Part model, mm, in its own coordinate system. A direction names the side the tool comes from. Round coordinates to 2 decimals unless told otherwise and drop trailing zeros. Write each loop counter-clockwise with the first axis right and the second up, starting at its lowest first coordinate (ties: lowest second). Pieces come first, ordered by that corner, then holes.
1) Which spindle directions (+Z, -Z, +X, -X, +Y, -Y) get a long thin tool onto all of the face, cutting with end or side? Do faces 1 (the cylindrical face through (-5.5, -24.9, 2.5)), 2 (the cylindrical face through (37.24, -20.517, 0.493)). Say none if no direction does.
2) Pull direction X, two halves, no side cores. Call faces 3 (the cylindrical face through (-43.93, -28.9, 0.99)), 4 (the cylindrical face through (43.93, 28.9, 0.99)), 5 (the cylindrical face through (-38.974, -21.148, 0.493)): +X half, -X half, draft (parallel to the pull), parting line (faces both ways), or undercut.
3) Saw through at B-B on y = 0. Write the cut outline in (x, z).
4) Saw through at A-A on x = -37.5. Write the cut outline in (y, z), and give its area (3 significant figures).
5) Flat gauge pin, fed straight in: pin 1 (8 mm diameter, centred on x = -35.5, y = 12.5, fed in from +Z). Where does the tip first touch, or does it go through?
6) Drill centre lines: L1, parallel to Y at x = 37.5, z = 0.7; L2, parallel to Y at x = 0, z = 0.9; L3, parallel to Z at x = -38, y = -17. Where is each one in solid material? Low to high.
7) Saw through at C-C on x = -3. Write the cut outline in (y, z), and give its area (3 significant figures).
8) Saw through at D-D on y = 22.5. Write the cut outline in (x, z), and give its area (3 significant figures).
```python
from build123d import *

# Parameters (mm, degrees)
SKETCH_R      = 20
SKETCH_R_2    = 2
PAD_DEPTH     = 2
SKETCH001_R   = 25.5
SKETCH001_R_2 = 25
PAD001_DEPTH  = 1
CHAMFER_SIZE  = 1


with BuildPart() as part:
    # Sketch → Pad (new body)
    with BuildSketch(Plane.XY):
        with BuildLine():
            Line((-42.5, 29.5), (42.5, 29.5))
            ThreePointArc((44.5, 27.5), (43.914214, 28.914214), (42.5, 29.5))
            Line((44.5, 27.5), (44.5, -27.5))
            ThreePointArc((42.5, -29.5), (43.914214, -28.914214), (44.5, -27.5))
            Line((42.5, -29.5), (-42.5, -29.5))
            ThreePointArc((-44.5, -27.5), (-43.914214, -28.914214), (-42.5, -29.5))
            Line((-44.5, -27.5), (-44.5, 27.5))
            ThreePointArc((-42.5, 29.5), (-43.914214, 28.914214), (-44.5, 27.5))
        make_face()
        Circle(SKETCH_R, mode=Mode.SUBTRACT)
        with Locations((-37.5, 22.5)):
            Circle(SKETCH_R_2, mode=Mode.SUBTRACT)
        with Locations((-37.5, -22.5)):
            Circle(SKETCH_R_2, mode=Mode.SUBTRACT)
        with Locations((37.5, 22.5)):
            Circle(SKETCH_R_2, mode=Mode.SUBTRACT)
        with Locations((37.5, -22.5)):
            Circle(SKETCH_R_2, mode=Mode.SUBTRACT)
    extrude(amount=PAD_DEPTH)

    # Sketch001 → Pad001 (join)
    with BuildSketch(Plane.XY.offset(2)):
        Circle(SKETCH001_R)
        Circle(SKETCH001_R_2, mode=Mode.SUBTRACT)
    extrude(amount=PAD001_DEPTH)

    # Chamfer
    chamfer_edges = [part.edges().sort_by_distance(p)[0] for p in [
        (-39.5, 22.5, 2),
        (-39.5, -22.5, 2),
        (35.5, 22.5, 2),
        (35.5, -22.5, 2),
    ]]
    chamfer(chamfer_edges, length=CHAMFER_SIZE)


solid = part.part
```
Completed:
1. face 1: +Z
1. face 2: +Z, -Z
2. face 3: -X half
2. face 4: +X half
2. face 5: undercut
3. outline: (-44.5, 0) - (-20, 0) - (-20, 2) - (-25, 2) - (-25, 3) - (-25.5, 3) - (-25.5, 2) - (-44.5, 2) - close; (20, 0) - (44.5, 0) - (44.5, 2) - (25.5, 2) - (25.5, 3) - (25, 3) - (25, 2) - (20, 2) - close
4. outline: (-29.5, 0) - (-24.5, 0) - (-24.5, 1) - (-25.5, 2) - (-29.5, 2) - close; (-20.5, 0) - (20.5, 0) - (20.5, 1) - (19.5, 2) - (-19.5, 2) - (-20.5, 1) - close; (24.5, 0) - (29.5, 0) - (29.5, 2) - (25.5, 2) - (24.5, 1) - close
4. area: 100 mm2
5. pin 1: stops at z = 2
6. L1: y = -29.5 to -24.5, -20.5 to 20.5, 24.5 to 29.5
6. L2: y = -29.5 to -20, 20 to 29.5
6. L3: z = 0 to 2
7. outline: (-29.5, 0) - (-19.77, 0) - (-19.77, 2) - (-24.82, 2) - (-24.82, 3) - (-25.32, 3) - (-25.32, 2) - (-29.5, 2) - close; (19.77, 0) - (29.5, 0) - (29.5, 2) - (25.32, 2) - (25.32, 3) - (24.82, 3) - (24.82, 2) - (19.77, 2) - close
7. area: 39.9 mm2
8. outline: (-44.5, 0) - (-39.5, 0) - (-39.5, 1) - (-40.5, 2) - (-44.5, 2) - close; (-35.5, 0) - (35.5, 0) - (35.5, 1) - (34.5, 2) - (12, 2) - (12, 3) - (10.9, 3) - (10.9, 2) - (-10.9, 2) - (-10.9, 3) - (-12, 3) - (-12, 2) - (-34.5, 2) - (-35.5, 1) - close; (39.5, 0) - (44.5, 0) - (44.5, 2) - (40.5, 2) - (39.5, 1) - close
8. area: 162 mm2
